The model under review builds one solid part; all positions refer to its coordinate system, in mm. A direction names the side the tool comes from. Round coordinates to 2 decimals unless told otherwise and drop trailing zeros. Write each loop counter-clockwise with the first axis right and the second up, starting at its lowest first coordinate (ties: lowest second). Pieces come first, ordered by that corner, then holes.
Item 1: Add section D-D (x = -14.5). Give the boundary of the cut face in (y, z).
Item 2: To check wall thickness, follow L1, parallel to Z at x = 0, y = 62.5; L2, parallel to Y at x = 6.5, z = 110; L3, parallel to Z at x = 14, y = 7. State the ranges of each line that lie inside material, in increasing order.
Item 3: Add section B-B (y = 7.5). Give the boundary of the cut face in (x, z), plus the area to 3 significant figures.
Item 4: Clearance check with flat-ended pins moving along their axes: pin 1 Ø12 at (x, z) = (0, 96.45) entering from -Y; pin 2 Ø23.5 at (x, z) = (-5.5, 90.5) entering from -Y. State where each tip first meets the part, or that it passes through.
Item 5: Draft analysis for pull direction Z (two halves, no side actions). For faces 1 (the face through (18, 0, 114)), 2 (the face through (0, 86, 126.454)), 3 (the face through (0.42, 8.51, 70.76)), state which applies: +Z half, -Z half, draft (parallel to the pull), parting line (faces both ways), or undercut.
Item 6: Machinability: for faces 4 (the face through (18, 0, 79)), 5 (the face through (0, 14, 107)), which of the approach directions +Z, -Z, +X, -X, +Y, -Y give a long, thin tool a straight path to every point of the face, cutting with its end or side? Answer none if there is none.
Item 7: Add section A-A (x = -2.5). Give the boundary of the cut face in (y, z).
Item 8: Add section C-C (z = 99). Give the boundary of the cut face in (x, y), plus the area to 3 significant figures.
```python
from build123d import *

# Parameters (mm, degrees)
SKETCH_1_W                = 160
SKETCH_1_H                = 60
EXTRUDE_1_DEPTH           = 60
HOLE_WIZARD_6_7_6_7_1_D   = 6.7
HOLE_WIZARD_1_D           = 20
HOLE_WIZARD_1_CBORE_D     = 47
HOLE_WIZARD_1_CBORE_DEPTH = 14
CHAMFER_1_SIZE            = 10


with BuildPart() as part:
    # Эскиз1 → Бобышка-Вытянуть1 (new body)
    with BuildSketch(Plane(origin=(-30, 0, 0), x_dir=(0, -1, 0), z_dir=(-1, 0, 0))):
        with Locations((-80, 96.453617418)):
            Rectangle(SKETCH_1_W, SKETCH_1_H)
    extrude(amount=-EXTRUDE_1_DEPTH)

    # Диаметр отверстия Ø6.7 (6.7)1 (through all)
    with Locations(Plane.ZY.offset(30)):
        with Locations((73.953617418, 7.5)):
            Hole(HOLE_WIZARD_6_7_6_7_1_D / 2)

    # Отверстие1 (through all)
    with Locations(Plane(origin=(0, 0, 0), x_dir=(-1, 0, 0), z_dir=(0, -1, 0))):
        with Locations((0, -96.453617418)):
            CounterBoreHole(HOLE_WIZARD_1_D / 2, HOLE_WIZARD_1_CBORE_D / 2, HOLE_WIZARD_1_CBORE_DEPTH)

    # Фаска1
    # the kernel refuses this chamfer: 10 mm, written as the material it takes off along each edge
    with BuildSketch(Plane(origin=(-30, 0, 40.736787538), x_dir=(0.9996219169112968, -0.027495876610586372, 0), z_dir=(0, 0, 1)), Plane(origin=(-55.71682988, 0, 126.453617418), x_dir=(0, -0.027495876610586372, -0.9996219169112968), z_dir=(1, 0, 0))) as chamfer_1_piece_1:
        Polygon((CHAMFER_1_SIZE * 0.999621916911, CHAMFER_1_SIZE * 0.0274958766106), (-CHAMFER_1_SIZE * 0.0274958766106, CHAMFER_1_SIZE * 0.999621916911), (0, 0), align=None)
    extrude(amount=111.433659759, mode=Mode.SUBTRACT)
    with BuildSketch(Plane(origin=(-55.71682988, 0, 66.453617418), x_dir=(0, -0.027495876610586372, 0.9996219169112968), z_dir=(1, 0, 0)), Plane(origin=(30, 0, 40.736787538), x_dir=(-0.9996219169112968, -0.027495876610586372, 0), z_dir=(0, 0, 1))) as chamfer_1_piece_2:
        Polygon((CHAMFER_1_SIZE * 0.999621916911, -CHAMFER_1_SIZE * 0.0274958766106), (-CHAMFER_1_SIZE * 0.0274958766106, -CHAMFER_1_SIZE * 0.999621916911), (0, 0), align=None)
    extrude(amount=111.433659759, mode=Mode.SUBTRACT)


solid = part.part
```
Numbers:
1. outline: (0, 76.45) - (10, 66.45) - (160, 66.45) - (160, 126.45) - (10, 126.45) - (0, 116.45) - (0, 114.95) - (14, 114.95) - (14, 77.96) - (0, 77.96) - close; hole circle Ø6.7 at (7.5, 73.95)
2. L1: z = 66.45 to 86.45, 106.45 to 126.45
2. L2: y = 14 to 160
2. L3: z = 69.45 to 70.64, 77.27 to 77.58, 115.33 to 123.45
3. outline: (-27.5, 68.95) - (27.5, 68.95) - (27.5, 70.6) - (-27.5, 70.6) - close; (-27.5, 77.3) - (-13.62, 77.3) arc R23.5 cw (long way) to (13.62, 77.3) - (27.5, 77.3) - (27.5, 123.95) - (-27.5, 123.95) - close
3. area: 1,000 mm2
4. pin 1: passes through
4. pin 2: stops at y = 14
5. face 1: draft
5. face 2: +Z half
5. face 3: undercut
6. face 4: +Z, -Z, +X, -X, -Y
6. face 5: -Y
7. outline: (3.37, 73.09) - (10, 66.45) - (160, 66.45) - (160, 86.77) - (14, 86.77) - (14, 73.09) - (10.74, 73.09) arc R3.35 cw to (4.26, 73.09) - close; (3.37, 119.82) - (14, 119.82) - (14, 106.14) - (160, 106.14) - (160, 126.45) - (10, 126.45) - close
8. outline: (-30, 10) - (-23.36, 3.36) - (-23.36, 14) - (-9.67, 14) - (-9.67, 160) - (-30, 160) - close; (9.67, 14) - (23.36, 14) - (23.36, 3.36) - (30, 10) - (30, 160) - (9.67, 160) - close
8. area: 6,030 mm2
